```python
from build123d import *
from build123d.topology import SkipClean

# Parameters (mm, degrees)
BASPROSKE_W         = 14
BASPROSKE_H         = 15
TOOTHCUT_DEPTH      = 26.416530054
TEETHCUTS_COUNT     = 10
TEETHCUTS_ANGLE     = 324
BORSKE_R            = 5
BORE_DEPTH          = 50.0005588
CUT_EXTRUDE1_DEPTH  = 26.09062294
BOSS_EXTRUDE1_DEPTH = 6


with BuildPart() as part:
    # BasProSke → Base-Revolve (revolve)
    with BuildSketch(Plane(origin=(0, 0, 0), x_dir=(1, 0, 0), z_dir=(0, 1, 0)), mode=Mode.PRIVATE) as base_revolve_sk:
        with Locations((7, 7.5)):
            Rectangle(BASPROSKE_W, BASPROSKE_H)
    revolve(base_revolve_sk.sketch.rotate(Axis((-10, 0, 0), (1, 0, 0)), 180), axis=Axis((-10, 0, 0), (1, 0, 0)))

    # TooCutSke → ToothCut (cut, through all)
    with BuildSketch(Plane(origin=(0, 0, 0), x_dir=(0, 0, -1), z_dir=(1, 0, 0))):
        with BuildLine():
            ThreePointArc((1.691642647, 9.220098761), (0, 9.374), (-1.691642647, 9.220098761))
            ThreePointArc((-1.691642647, 9.220098761), (-2.059354944, 12.219114282), (-4.087513468, 14.458730194))
            ThreePointArc((-4.087513468, 14.458730194), (0, 15.0254), (4.087513468, 14.458730194))
            ThreePointArc((4.087513468, 14.458730194), (2.059354944, 12.219114282), (1.691642647, 9.220098761))
        make_face()
    toothcut = extrude(amount=TOOTHCUT_DEPTH, mode=Mode.SUBTRACT)

    # TeethCuts: ToothCut ×10 about axis
    teethcuts_axis = Axis((-10, 0, 0), (1, 0, 0))
    for i in range(1, TEETHCUTS_COUNT):
        add(toothcut.rotate(teethcuts_axis, i * TEETHCUTS_ANGLE / (TEETHCUTS_COUNT - 1)), mode=Mode.SUBTRACT)

    # BorSke → Bore (cut, symmetric)
    with BuildSketch(Plane(origin=(0, 0, 0), x_dir=(0, 0, -1), z_dir=(1, 0, 0))):
        with Locations(Location((0, 0, 0), (0, 0, 180))):
            Circle(BORSKE_R)
    extrude(amount=BORE_DEPTH, both=True, mode=Mode.SUBTRACT)

    # Sketch1 → Cut-Extrude1 (cut, through all)
    with BuildSketch(Plane(origin=(14, 0, 0), x_dir=(0, 0, -1), z_dir=(1, 0, 0))):
        Polygon((0, -7.332348419), (6.35, -3.666174209), (6.35, 3.666174209), (0, 7.332348419), (-6.35, 3.666174209), (-6.35, -3.666174209), align=None)
    extrude(amount=-CUT_EXTRUDE1_DEPTH, mode=Mode.SUBTRACT)

    # Sketch2 → Boss-Extrude1 (add)
    with SkipClean():  # the faces are left unmerged after this step: merging them gives an invalid solid
        with BuildSketch(Plane(origin=(14, 0, 0), x_dir=(0, 0, -1), z_dir=(1, 0, 0))):
            with BuildLine():
                ThreePointArc((14.987839303, -0.603881639), (15, 0), (14.987839303, 0.603881639))
                ThreePointArc((14.987839303, 0.603881639), (12.239957624, 1.819335924), (9.291581333, 1.240319444))
                ThreePointArc((9.291581333, 1.240319444), (8.915203784, 2.896725305), (8.246088681, 4.45801497))
                ThreePointArc((8.246088681, 4.45801497), (10.971712553, 5.7225929), (12.480369426, 8.321080397))
                ThreePointArc((12.480369426, 8.321080397), (12.135254916, 8.816778784), (11.770463983, 9.298181415))
                ThreePointArc((11.770463983, 9.298181415), (8.832954904, 8.666340261), (6.788005726, 6.464893987))
                ThreePointArc((6.788005726, 6.464893987), (5.509898955, 7.583725305), (4.050870426, 8.453539187))
                ThreePointArc((4.050870426, 8.453539187), (5.512646202, 11.078685739), (5.205822621, 14.067672545))
                ThreePointArc((5.205822621, 14.067672545), (4.635254916, 14.265847744), (4.057171486, 14.440891923))
                ThreePointArc((4.057171486, 14.440891923), (2.052063631, 12.203097177), (1.691642647, 9.220098761))
                ThreePointArc((1.691642647, 9.220098761), (0, 9.374), (-1.691642647, 9.220098761))
                ThreePointArc((-1.691642647, 9.220098761), (-2.052063631, 12.203097177), (-4.057171486, 14.440891923))
                ThreePointArc((-4.057171486, 14.440891923), (-4.635254916, 14.265847744), (-5.205822621, 14.067672545))
                ThreePointArc((-5.205822621, 14.067672545), (-5.512646202, 11.078685739), (-4.050870426, 8.453539187))
                ThreePointArc((-4.050870426, 8.453539187), (-5.509898955, 7.583725305), (-6.788005726, 6.464893987))
                ThreePointArc((-6.788005726, 6.464893987), (-8.832954904, 8.666340261), (-11.770463983, 9.298181415))
                ThreePointArc((-11.770463983, 9.298181415), (-12.135254916, 8.816778784), (-12.480369426, 8.321080397))
                ThreePointArc((-12.480369426, 8.321080397), (-10.971712553, 5.7225929), (-8.246088681, 4.45801497))
                ThreePointArc((-8.246088681, 4.45801497), (-8.915203784, 2.896725305), (-9.291581333, 1.240319444))
                ThreePointArc((-9.291581333, 1.240319444), (-12.239957624, 1.819335924), (-14.987839303, 0.603881639))
                ThreePointArc((-14.987839303, 0.603881639), (-15, 0), (-14.987839303, -0.603881639))
                ThreePointArc((-14.987839303, -0.603881639), (-12.239957624, -1.819335924), (-9.291581333, -1.240319444))
                ThreePointArc((-9.291581333, -1.240319444), (-8.915203784, -2.896725305), (-8.246088681, -4.45801497))
                ThreePointArc((-8.246088681, -4.45801497), (-10.971712553, -5.7225929), (-12.480369426, -8.321080397))
                ThreePointArc((-12.480369426, -8.321080397), (-12.135254916, -8.816778784), (-11.770463983, -9.298181415))
                ThreePointArc((-11.770463983, -9.298181415), (-8.832954904, -8.666340261), (-6.788005726, -6.464893987))
                ThreePointArc((-6.788005726, -6.464893987), (-5.509898955, -7.583725305), (-4.050870426, -8.453539187))
                ThreePointArc((-4.050870426, -8.453539187), (-5.512646202, -11.078685739), (-5.205822621, -14.067672545))
                ThreePointArc((-5.205822621, -14.067672545), (-4.635254916, -14.265847744), (-4.057171486, -14.440891923))
                ThreePointArc((-4.057171486, -14.440891923), (-2.052063631, -12.203097177), (-1.691642647, -9.220098761))
                ThreePointArc((-1.691642647, -9.220098761), (0, -9.374), (1.691642647, -9.220098761))
                ThreePointArc((1.691642647, -9.220098761), (2.052063631, -12.203097177), (4.057171486, -14.440891923))
                ThreePointArc((4.057171486, -14.440891923), (4.635254916, -14.265847744), (5.205822621, -14.067672545))
                ThreePointArc((5.205822621, -14.067672545), (5.512646202, -11.078685739), (4.050870426, -8.453539187))
                ThreePointArc((4.050870426, -8.453539187), (5.509898955, -7.583725305), (6.788005726, -6.464893987))
                ThreePointArc((6.788005726, -6.464893987), (8.832954904, -8.666340261), (11.770463983, -9.298181415))
                ThreePointArc((11.770463983, -9.298181415), (12.135254916, -8.816778784), (12.480369426, -8.321080397))
                ThreePointArc((12.480369426, -8.321080397), (10.971712553, -5.7225929), (8.246088681, -4.45801497))
                ThreePointArc((8.246088681, -4.45801497), (8.915203784, -2.896725305), (9.291581333, -1.240319444))
                ThreePointArc((9.291581333, -1.240319444), (12.239957624, -1.819335924), (14.987839303, -0.603881639))
            make_face()
            Polygon((-6.35, -3.666174209), (0, -7.332348419), (6.35, -3.666174209), (6.35, 3.666174209), (0, 7.332348419), (-6.35, 3.666174209), align=None, mode=Mode.SUBTRACT)
        extrude(amount=BOSS_EXTRUDE1_DEPTH)


solid = part.part
```
Geometry: final body of the model. Coordinates: model frame, mm. A direction names the side the tool comes from. Coordinates: 2 decimals unless noted, no trailing zeros. Order: outer loops, then holes, each group sorted by start corner. A loop starts at its lowest first (then second) coordinate and runs counter-clockwise, first axis right, second up.
Item 1: Section query B-B (z = -2.5). Output: boundary loops of the cut face in (x, y).
Answer:
outline: (0, -12.99) - (20, -12.99) - (20, -5.89) - (0, -5.89) - close; (0, 5.89) - (20, 5.89) - (20, 12.99) - (0, 12.99) - close
Item 2: Contact query for flat-ended pins moving along their axis: P1, Ø5, axis at x = 14, y = -6.5, coming from the -Z side; P2, Ø5, axis at x = 15, y = 10.5, coming from the +Z side; P3, Ø2, axis at x = 11.5, z = -11.5, coming from the -Y side. Output: stop coordinate, or through.
Answer:
P1: stops at z = -12.48
P2: stops at z = 12.48
P3: stops at y = -9.32
Item 3: Section query A-A (y = -12.5). Output: boundary loops of the cut face in (x, z).
Answer:
outline: (0, -5.6) - (20, -5.6) - (20, -2.2) - (0, -2.2) - close; (0, 2.2) - (20, 2.2) - (20, 5.6) - (0, 5.6) - close
Item 4: Section query C-C (z = 10). Output: boundary loops of the cut face in (x, y).
Answer:
outline: (0, -9.15) - (20, -9.15) - (20, -5.03) - (0, -5.03) - close; (0, -1.56) - (20, -1.56) - (20, 1.56) - (0, 1.56) - close; (0, 5.03) - (20, 5.03) - (20, 9.15) - (0, 9.15) - close
Item 5: Access query for faces 3 (the face through (9.86, 5.474, -3.219)), 4 (the face through (0, 0, 7)). Directions: +Z, -Z, +X, -X, +Y, -Y. A direction counts if a zero-diameter tool reaches every point of the face in a straight line with its end or side. Return the directions, or none.
Answer:
face 3: +X, -X
face 4: +Z, -Z, -X, +Y, -Y
Item 6: Material intervals for line 1 along Y through (x, z) = (7.5, -4.5); line 2 along Z through (x, y) = (14.75, 0.25); line 3 along Z through (x, y) = (12, -8), sorted ascending.
Answer:
line 1: y = -14.31 to -8.94, -8.22 to -4.73, 4.73 to 8.22, 8.94 to 14.31
line 2: z = -15 to -6.35, 6.35 to 15
line 3: z = -12.4 to -7.92, -4.89 to 4.89, 7.92 to 12.4
Item 7: Draft query along Z for faces 1 (the face through (20, 0.2, -6.5)), 2 (the face through (9.86, -9.374, 0.024)). Return one class per face: released by +Z, released by -Z, zero draft, split by the parting line, or undercut.
Answer:
face 1: zero draft
face 2: undercut
Item 8: Section query D-D (y = 10.25). Output: boundary loops of the cut face in (x, z).
Answer:
outline: (0, -5.27) - (20, -5.27) - (20, -1.61) - (0, -1.61) - close; (0, 1.61) - (20, 1.61) - (20, 5.27) - (0, 5.27) - close
